Part print with two shaded views. Sizes in mm from the minimum x, y, z corner. A direction names the side the tool comes from. Give positions to 0.01 mm unless a question says otherwise; leave off trailing zeros. Loops run counter-clockwise (first coordinate to the right, second up) from the corner with the lowest first, then second, coordinate; pieces in that order, holes last. Notation, with made-up numbers: (25, 25) -> (37, 25) arc R24 ccw to (37, 59) -> close; hole circle Ø5 at (86.25, 4). An arc over 180 degrees is marked (long way). One line per question, with ' | ' between items. Start each with the question number.
(1) Mould opens along X. For the marked faces 3, 4 and 5 say: pulls with the +X half, pulls with the -X half, needs draft (parallel to the pull), parting line crosses it, or undercut.
(2) Slice it at D-D, the plane x = 4.05. Write the cut outline in (y, z).
(3) Slice it at B-B, the plane z = 8.5. Write the cut outline in (x, y).
(4) Flat gauge pins, fed straight in: pin 1 Ø1.5 at (x, y) = (1.5, 0.5) entering from -Z; pin 2 Ø0.6 at (x, y) = (2, 2.5) entering from +Z; pin 3 Ø1 at (y, z) = (2, 11) entering from -X. Where does each tip first touch, or does it go through?
(5) Drill centre lines: L1, parallel to Z at x = 0.4, y = 3.3; L2, parallel to X at y = 1.5, z = 4.75; L3, parallel to Y at x = 2.2, z = 9.5. Where is each one in solid material? Low to high. Write a range as from..to.
(6) Slice it at C-C, the plane y = 4.2. Write the cut outline in (x, z).
(7) Slice it at A-A, the plane x = 2.25. Write the cut outline in (y, z).
(8) 3-axis set-ups, long thin cutter, end or side, ignore diameter. For the marked faces 1 and 2: which of +Z, -Z, +X, -X, +Y, -Y reach the whole face in a straight line?
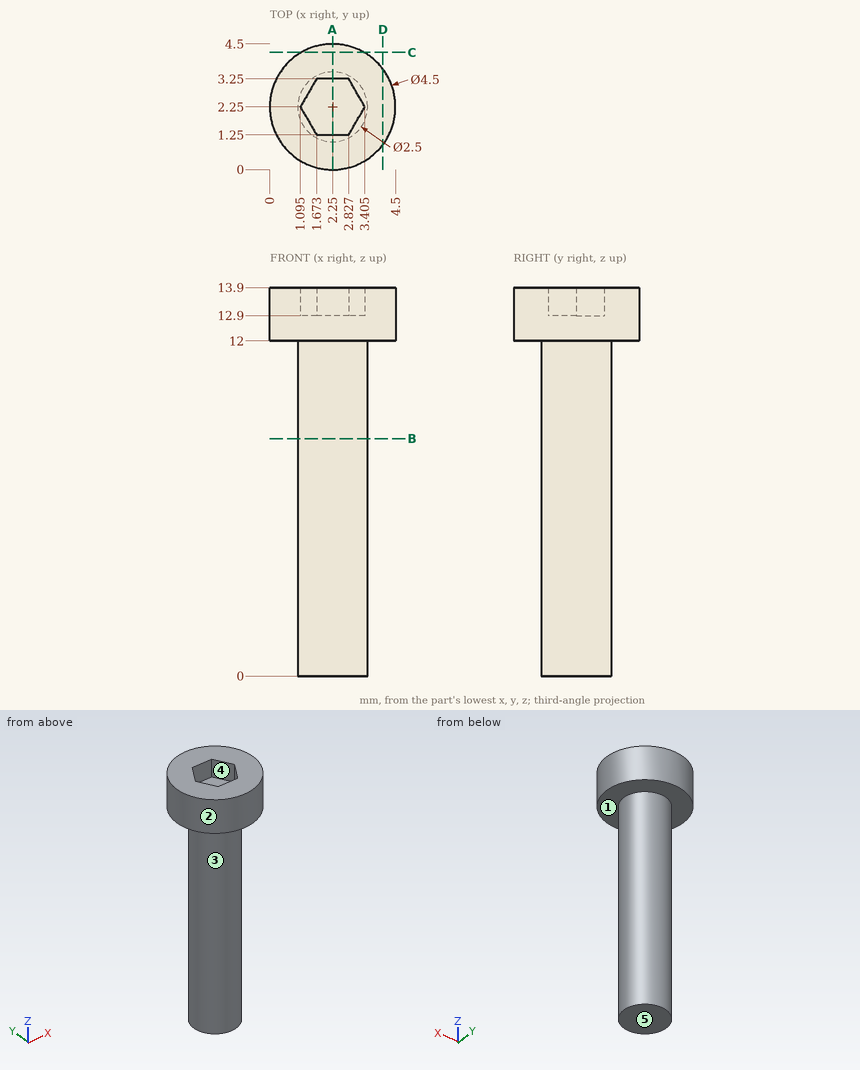
Final values:
1) face 3: parting line crosses it | face 4: undercut | face 5: needs draft
2) outline: (0.9, 12) -> (3.6, 12) -> (3.6, 13.9) -> (0.9, 13.9) -> close
3) outline: circle Ø2.5 at (2.25, 2.25)
4) pin 1: z = 0 | pin 2: z = 12.9 | pin 3: x = 1
5) L1: 12..13.9 | L2: 1.25..3.25 | L3: 1..3.5
6) outline: (1.13, 12) -> (3.37, 12) -> (3.37, 13.9) -> (1.13, 13.9) -> close
7) outline: (0, 12) -> (1, 12) -> (1, 0) -> (3.5, 0) -> (3.5, 12) -> (4.5, 12) -> (4.5, 13.9) -> (3.25, 13.9) -> (3.25, 12.9) -> (1.25, 12.9) -> (1.25, 13.9) -> (0, 13.9) -> close
8) face 1: -Z | face 2: +Z, -Z
